Source: three-view drawing plus pictorial views. Frame: mm from the lowest corner of the part. A direction names the side the tool comes from. Coordinates: 2 decimals unless noted, no trailing zeros. Write each loop counter-clockwise with the first axis right and the second up, starting at its lowest first coordinate (ties: lowest second). Pieces come first, ordered by that corner, then holes. Notation, with made-up numbers: (60, 36.25) - (65, 36.25) arc R14 ccw to (65, 52.25) - close; hole circle Ø2 at (25.5, -31). An arc over 180 degrees is marked (long way). One line per item, written item: value.
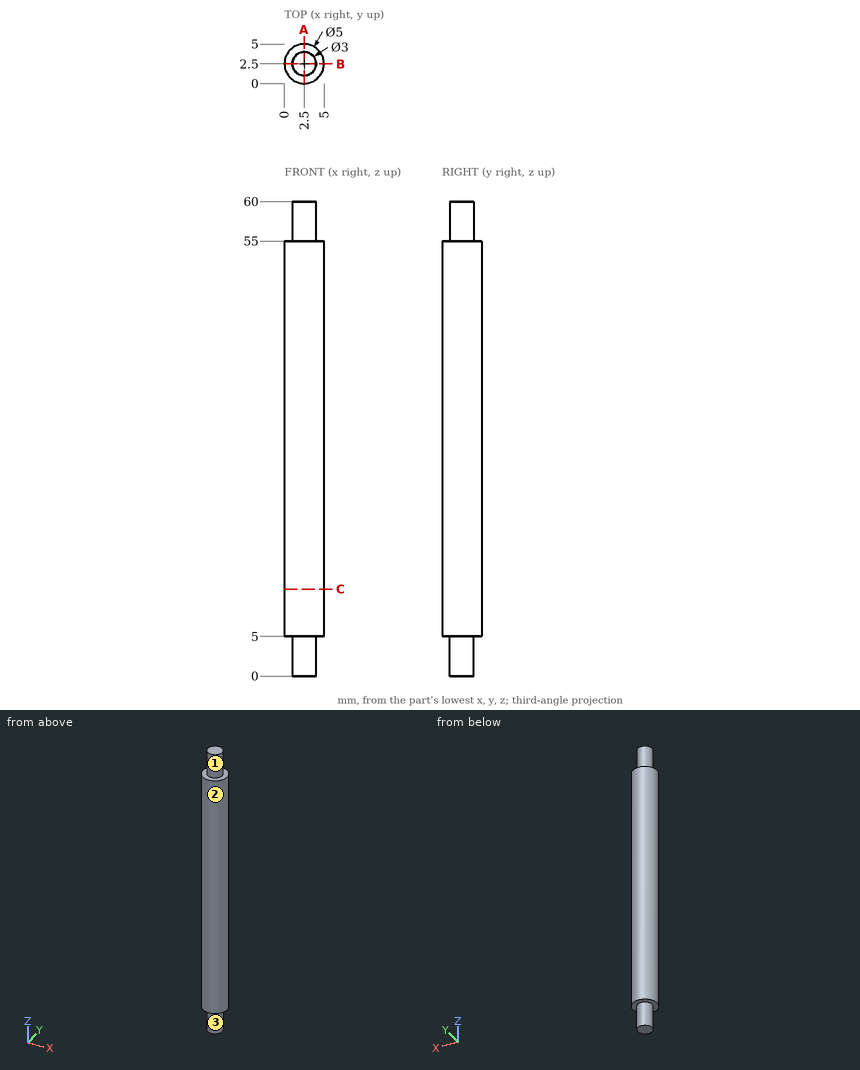
1) Reachability of the marked faces 1, 2 and 3 from +Z, -Z, +X, -X, +Y, -Y: full face, straight path, thin tool, end or side. Return the list, or none.
Values found:
face 1: +Z
face 2: +Z, -Z
face 3: -Z
2) Section query A-A on x = 2.5. Output: boundary loops of the cut face in (y, z).
Values found:
outline: (0, 5) - (1, 5) - (1, 0) - (4, 0) - (4, 5) - (5, 5) - (5, 55) - (4, 55) - (4, 60) - (1, 60) - (1, 55) - (0, 55) - close
3) Contact query for flat-ended pins moving along their axis: P1, Ø1, axis at y = 3.5, z = 41, coming from the +X side; P2, Ø1.5, axis at y = 3.5, z = 35.5, coming from the -X side. Output: stop coordinate, or through.
Values found:
P1: x = 4.95
P2: x = 0.01
4) Material intervals for line 1 (Z direction, x = 4.35, y = 1.4); line 2 (Y direction, x = 2.35, z = 9); line 3 (Y direction, x = 4.5, z = 12.5), sorted ascending.
Values found:
line 1: 5 to 55
line 2: 0 to 5
line 3: 1 to 4
5) Section query C-C on z = 11. Output: boundary loops of the cut face in (x, y), then the cut area to 3 significant figures.
Values found:
outline: circle Ø5 at (2.5, 2.5)
area: 19.6 mm2
